```python
from build123d import *

# Parameters (mm, degrees)
ESQUISSE2_W                               = 40
ESQUISSE2_H                               = 10
BOSS_EXTRU_1_DEPTH                        = 40
DIAM_TRE_DU_PER_AGE_4_1_4_1_1_D           = 4.1
TROU_POUR_TARAUDAGE_POUR_TROU_TARAUD_M3_D = 2.5
CHANFREIN1_SIZE                           = 0.5
R_P_TITION_LIN_AIRE2_COUNT                = 2
R_P_TITION_LIN_AIRE2_PITCH                = 10
ENL_V_START                               = 8
ESQUISSE20_R                              = 30.056093749
ENL_V_MAT_EXTRU_1_DEPTH                   = 1.6
R_P_TITION_LIN_AIRE1_COUNT                = 8
R_P_TITION_LIN_AIRE1_PITCH                = 3.2


with BuildPart() as part:
    # Esquisse2 → Boss.-Extru.1 (new body)
    with BuildSketch(Plane.XY):
        with Locations((20, 5)):
            Rectangle(ESQUISSE2_W, ESQUISSE2_H)
    extrude(amount=BOSS_EXTRU_1_DEPTH)

    # Diamètre du perçage Ø4.1 (4.1)1 (through all)
    with Locations(Plane.XY.offset(40)):
        with Locations((25, 5)):
            diam_tre_du_per_age_4_1_4_1_1 = Hole(DIAM_TRE_DU_PER_AGE_4_1_4_1_1_D / 2)

    # Esquisse9 → Trou pour taraudage pour trou taraudé M61 (revolve, cut)
    with BuildSketch(Plane(origin=(25, 5, 40), x_dir=(0, -1, 0), z_dir=(1, 0, 0))):
        Polygon((0, 0), (0, 9.502151548), (2.5, 8), (2.5, 0), align=None)
    trou_pour_taraudage_pour_trou_taraud_m6 = revolve(axis=Axis((25, 5, 46.35), (0, 0, -1)), mode=Mode.SUBTRACT)

    # Esquisse13 → Diamètre du perçage Ø6.0 (6)1 (revolve, cut)
    with BuildSketch(Plane(origin=(25, 5, 0), x_dir=(0, 1, 0), z_dir=(1, 0, 0))):
        Polygon((0, 0), (0, 21.802581857), (3, 20), (3, 0), align=None)
    diam_tre_du_per_age_6_0_6_1 = revolve(axis=Axis((25, 5, -6.35), (0, 0, 1)), mode=Mode.SUBTRACT)

    # Trou pour taraudage pour trou taraud_ M3 (through all)
    with Locations(Plane(origin=(0, 0, 0), x_dir=(-1, 0, 0), z_dir=(0, -1, 0))):
        with Locations((-4, -36), (-36, -36), (-36, -4), (-4, -4)):
            Hole(TROU_POUR_TARAUDAGE_POUR_TROU_TARAUD_M3_D / 2)

    # Esquisse18 → Trou pour taraudage pour trou taraud 2 (revolve, cut)
    with BuildSketch(Plane(origin=(25, 0, 4), x_dir=(0, 0, -1), z_dir=(1, 0, 0))):
        Polygon((0, 0), (0, 5.751075774), (1.25, 5), (1.25, 0), align=None)
    trou_pour_taraudage_pour_trou_taraud_2 = revolve(axis=Axis((25, -6.35, 4), (0, 1, 0)), mode=Mode.SUBTRACT)

    # Chanfrein1
    chanfrein1_edges = [part.edges().sort_by_distance(p)[0] for p in [
        (40, 5, 40),
        (20, 10, 40),
        (0, 5, 40),
        (20, 10, 0),
        (40, 5, 0),
        (20, 0, 0),
        (0, 5, 0),
        (20, 0, 40),
        (0, 10, 20),
        (40, 10, 20),
        (40, 0, 20),
        (0, 0, 20),
    ]]
    chamfer(chanfrein1_edges, length=CHANFREIN1_SIZE)

    # Répétition linéaire2: Diamètre du perçage Ø4.1 (4.1)1, Trou pour taraudage pour trou taraudé M61, Diamètre du perçage Ø6.0 (6)1, Trou pour taraudage pour trou taraud 2 ×2
    with Locations(*[(-i * R_P_TITION_LIN_AIRE2_PITCH, 0, 0) for i in range(1, R_P_TITION_LIN_AIRE2_COUNT)]):
        add(diam_tre_du_per_age_4_1_4_1_1, mode=Mode.SUBTRACT)
        add(trou_pour_taraudage_pour_trou_taraud_m6, mode=Mode.SUBTRACT)
        add(diam_tre_du_per_age_6_0_6_1, mode=Mode.SUBTRACT)
        add(trou_pour_taraudage_pour_trou_taraud_2, mode=Mode.SUBTRACT)

    # Esquisse20 → Enlèv. mat.-Extru.1 (cut)
    with BuildSketch(Plane(origin=(0, 40, 40), x_dir=(-1, 0, 0), z_dir=(0, 0, -1)).offset(ENL_V_START)):
        with Locations((-20, -35)):
            Circle(ESQUISSE20_R)
        with BuildLine():
            Line((-15, -40), (-25, -40))
            ThreePointArc((-25, -40), (-30, -35), (-25, -30))
            Line((-25, -30), (-15, -30))
            ThreePointArc((-15, -30), (-10, -35), (-15, -40))
        make_face(mode=Mode.SUBTRACT)
    enl_v_mat_extru_1 = extrude(amount=ENL_V_MAT_EXTRU_1_DEPTH, mode=Mode.SUBTRACT)

    # Répétition linéaire1: Enlèv. mat.-Extru.1 ×8
    with Locations(*[(0, 0, -i * R_P_TITION_LIN_AIRE1_PITCH) for i in range(1, R_P_TITION_LIN_AIRE1_COUNT)]):
        add(enl_v_mat_extru_1, mode=Mode.SUBTRACT)


solid = part.part
```
The listing builds one solid part. Answer for the finished solid, in the listing's coordinates (mm). A direction names the side the tool comes from. Coordinates: 2 decimals unless noted, no trailing zeros. Loops run counter-clockwise (first coordinate to the right, second up) from the corner with the lowest first, then second, coordinate; pieces in that order, holes last. Notation, with made-up numbers: (42.5, -5) -> (62.5, -5) arc R12 ccw to (62.5, 6) -> close; hole circle Ø2 at (-11, 32). An arc over 180 degrees is marked (long way). Return JSON: item names as keys, results as strings. Group by question number.
(1) A cutting plane is placed at C-C on z = 26.5. Write down the section's boundary in (x, y).
(2) Find the intervals of material crossed by probe 1 along X at (y, z) = (5, 25); probe 2 along X at (y, z) = (1.6, 4); probe 3 along X at (y, z) = (5, 12), in increasing order. Write a range as from..to.
(3) Determine the mould class of faces 1 (the cylindrical face through (14.62, 1.12, 2.81)), 2 (the flat face through (40, 5, 23)), 3 (the flat face through (20, 10, 20)) for opening direction X: released by +X, released by -X, zero draft, split by the parting line, or undercut.
(4) Which of the six approach directions +Z, -Z, +X, -X, +Y, -Y give full straight-line access (tool end or side, diameter ignored) to faces 4 (the flat face through (40, 5, 26)), 5 (the cylindrical face through (30, 5, 12))?
(5) A cutting plane is placed at A-A on z = 36. Write down the section's boundary in (x, y), and give its area (3 significant figures).
(6) A cutting plane is placed at D-D on y = 4.25. Count the separate pieces of the cut face and the enclosed holes in it, and give its area (3 significant figures).
(7) A cutting plane is placed at B-B on z = 4. Write down the section's boundary in (x, y), and give its area (3 significant figures).
The answers:
{
 "1": {"outline": "(0, 0.5) -> (0.5, 0) -> (39.5, 0) -> (40, 0.5) -> (40, 9.5) -> (39.5, 10) -> (0.5, 10) -> (0, 9.5) -> close; hole circle Ø4.1 at (15, 5); hole circle Ø4.1 at (25, 5)"},
 "2": {"probe 1": "x = 10..12.95, 17.05..22.95, 27.05..30", "probe 2": "x = 0..2.75, 5.25..13.75, 16.25..23.75, 26.25..34.75, 37.25..40", "probe 3": "x = 10..12, 18..22, 28..30"},
 "3": {"face 1": "undercut", "face 2": "released by +X", "face 3": "zero draft"},
 "4": {"face 4": "+Z, -Z, +X, +Y, -Y", "face 5": "+X"},
 "5": {"outline": "(0, 0.5) -> (0.5, 0) -> (2.75, 0) -> (2.75, 10) -> (0.5, 10) -> (0, 9.5) -> close; (5.25, 0) -> (34.75, 0) -> (34.75, 10) -> (5.25, 10) -> close; (37.25, 0) -> (39.5, 0) -> (40, 0.5) -> (40, 9.5) -> (39.5, 10) -> (37.25, 10) -> close; hole circle Ø5 at (15, 5); hole circle Ø5 at (25, 5)", "area": "310 mm^2"},
 "6": {"separate pieces": "3", "enclosed holes": "4", "area": "921 mm^2"},
 "7": {"outline": "(0, 0.5) -> (0.5, 0) -> (2.75, 0) -> (2.75, 10) -> (0.5, 10) -> (0, 9.5) -> close; (5.25, 0) -> (13.75, 0) -> (13.75, 2.27) arc R3 cw (long way) to (16.25, 2.27) -> (16.25, 0) -> (23.75, 0) -> (23.75, 2.27) arc R3 cw (long way) to (26.25, 2.27) -> (26.25, 0) -> (34.75, 0) -> (34.75, 10) -> (5.25, 10) -> close; (37.25, 0) -> (39.5, 0) -> (40, 0.5) -> (40, 9.5) -> (39.5, 10) -> (37.25, 10) -> close", "area": "283 mm^2"}
}
